from build123d import *

# Parameters (mm, degrees)
F0_W      = 1200
F0_H      = 145
F1_DEPTH  = 22
F0_H_2    = 100
F2_W      = 145
F2_H      = 655
F2_H_2    = 145
F3_DEPTH  = 22
F4_W      = 145
F4_H      = 100
F6_DEPTH  = 78
F4_H_2    = 145
F5_W      = 145
F5_H      = 145
F5_H_2    = 100
F7_W      = 145
F7_H      = 100
F7_W_2    = 1055
F8_DEPTH  = 22
F7_W_3    = 1200
F7_H_2    = 145
F10_SIZE  = 15
F11_W     = 527.5
F11_H     = 145
F12_DEPTH = 211


# Not quite as in the source:
# - a feature names something its author has since deleted; it is built from what else it names


with BuildPart() as f1:
    # F0 (on Top) → F1 (new body)
    with BuildSketch(Plane.XY):
        with Locations((0, 327.5)):
            Rectangle(F0_W, F0_H)
    extrude(amount=-F1_DEPTH)


with BuildPart() as f1b:
    # F0 (on Top) → F1, piece 2 (new body)
    with BuildSketch(Plane.XY):
        with Locations((0, 163.75)):
            Rectangle(F0_W, F0_H_2)
    extrude(amount=-F1_DEPTH)


with BuildPart() as f1c:
    # F0 (on Top) → F1, piece 3 (new body)
    with BuildSketch(Plane.XY):
        Rectangle(F0_W, F0_H)
    extrude(amount=-F1_DEPTH)


with BuildPart() as f1d:
    # F0 (on Top) → F1, piece 4 (new body)
    with BuildSketch(Plane.XY):
        with Locations((0, -163.75)):
            Rectangle(F0_W, F0_H_2)
    extrude(amount=-F1_DEPTH)


with BuildPart() as f1e:
    # F0 (on Top) → F1, piece 5 (new body)
    with BuildSketch(Plane.XY):
        with Locations((0, -327.5)):
            Rectangle(F0_W, F0_H)
    extrude(amount=-F1_DEPTH)


with BuildPart() as f3:
    # F2 (on face) → F3 (new body)
    with BuildSketch(Plane(origin=(0, 0, -22), x_dir=(1, 0, 0), z_dir=(0, 0, -1))):
        with Locations((-527.5, -72.5)):
            Rectangle(F2_W, F2_H)
        with Locations((-527.5, 327.5)):
            Rectangle(F2_W, F2_H_2)
    extrude(amount=F3_DEPTH)


with BuildPart() as f3b:
    # F2 (on face) → F3, piece 2 (new body)
    with BuildSketch(Plane(origin=(0, 0, -22), x_dir=(1, 0, 0), z_dir=(0, 0, -1))):
        with Locations((0, 327.5)):
            Rectangle(F2_W, F2_H_2)
        with Locations((0, -72.5)):
            Rectangle(F2_W, F2_H)
    extrude(amount=F3_DEPTH)


with BuildPart() as f3c:
    # F2 (on face) → F3, piece 3 (new body)
    with BuildSketch(Plane(origin=(0, 0, -22), x_dir=(1, 0, 0), z_dir=(0, 0, -1))):
        with Locations((527.5, 327.5)):
            Rectangle(F2_W, F2_H_2)
        with Locations((527.5, -72.5)):
            Rectangle(F2_W, F2_H)
    extrude(amount=F3_DEPTH)


with BuildPart() as f6:
    # F4 (on face) → F6 (new body)
    with BuildSketch(Plane(origin=(0, 0, -44), x_dir=(1, 0, 0), z_dir=(0, 0, -1))):
        with Locations((-527.5, -350)):
            Rectangle(F4_W, F4_H)
    extrude(amount=F6_DEPTH)


with BuildPart() as f6b:
    # F4 (on face) → F6, piece 2 (new body)
    with BuildSketch(Plane(origin=(0, 0, -44), x_dir=(1, 0, 0), z_dir=(0, 0, -1))):
        with Locations((-527.5, 350)):
            Rectangle(F4_W, F4_H)
    extrude(amount=F6_DEPTH)


with BuildPart() as f6c:
    # F4 (on face) → F6, piece 3 (new body)
    with BuildSketch(Plane(origin=(0, 0, -44), x_dir=(1, 0, 0), z_dir=(0, 0, -1))):
        with Locations((527.5, -350)):
            Rectangle(F4_W, F4_H)
    extrude(amount=F6_DEPTH)


with BuildPart() as f6d:
    # F4 (on face) → F6, piece 4 (new body)
    with BuildSketch(Plane(origin=(0, 0, -44), x_dir=(1, 0, 0), z_dir=(0, 0, -1))):
        with Locations((527.5, 0)):
            Rectangle(F4_W, F4_H_2)
    extrude(amount=F6_DEPTH)


with BuildPart() as f6e:
    # F4 (on face) → F6, piece 5 (new body)
    with BuildSketch(Plane(origin=(0, 0, -44), x_dir=(1, 0, 0), z_dir=(0, 0, -1))):
        with Locations((527.5, 350)):
            Rectangle(F4_W, F4_H)
    extrude(amount=F6_DEPTH)


with BuildPart() as f6f:
    # F4 (on face) → F6, piece 6 (new body)
    with BuildSketch(Plane(origin=(0, 0, -44), x_dir=(1, 0, 0), z_dir=(0, 0, -1))):
        with Locations((-527.5, 0)):
            Rectangle(F4_W, F4_H_2)
    extrude(amount=F6_DEPTH)


with BuildPart() as f6g:
    # F5 (on face) → F6, piece 7 (new body)
    with BuildSketch(Plane(origin=(0, 0, -44), x_dir=(1, 0, 0), z_dir=(0, 0, -1))):
        Rectangle(F5_W, F5_H)
    extrude(amount=F6_DEPTH)


with BuildPart() as f6h:
    # F5 (on face) → F6, piece 8 (new body)
    with BuildSketch(Plane(origin=(0, 0, -44), x_dir=(1, 0, 0), z_dir=(0, 0, -1))):
        with Locations((0, 350)):
            Rectangle(F5_W, F5_H_2)
    extrude(amount=F6_DEPTH)


with BuildPart() as f6i:
    # F5 (on face) → F6, piece 9 (new body)
    with BuildSketch(Plane(origin=(0, 0, -44), x_dir=(1, 0, 0), z_dir=(0, 0, -1))):
        with Locations((0, -350)):
            Rectangle(F5_W, F5_H_2)
    extrude(amount=F6_DEPTH)


with BuildPart() as f8:
    # F7 (on face) → F8 (new body)
    with BuildSketch(Plane(origin=(0, 0, -122), x_dir=(1, 0, 0), z_dir=(0, 0, -1))):
        with Locations((-527.5, -350)):
            Rectangle(F7_W, F7_H)
        with Locations((72.5, -350)):
            Rectangle(F7_W_2, F7_H)
    extrude(amount=F8_DEPTH)


with BuildPart() as f8b:
    # F7 (on face) → F8, piece 2 (new body)
    with BuildSketch(Plane(origin=(0, 0, -122), x_dir=(1, 0, 0), z_dir=(0, 0, -1))):
        Rectangle(F7_W_3, F7_H_2)
    extrude(amount=F8_DEPTH)


with BuildPart() as f8c:
    # F7 (on face) → F8, piece 3 (new body)
    with BuildSketch(Plane(origin=(0, 0, -122), x_dir=(1, 0, 0), z_dir=(0, 0, -1))):
        with Locations((0, 350)):
            Rectangle(F7_W_3, F7_H)
    extrude(amount=F8_DEPTH)


with BuildPart() as f3c_1:
    add(f3c.part)

    # F9: union F3b, F3, F1, F1b, F1e, F1d, F1c, F6, F6b, F6d, F6f, F8b, F8c, F6e, F6c, F8, F6i, F6g, F6h
    add(f3b.part)
    add(f3.part)
    add(f1.part)
    add(f1b.part)
    add(f1e.part)
    add(f1d.part)
    add(f1c.part)
    add(f6.part)
    add(f6b.part)
    add(f6d.part)
    add(f6f.part)
    add(f8b.part)
    add(f8c.part)
    add(f6e.part)
    add(f6c.part)
    add(f8.part)
    add(f6i.part)
    add(f6g.part)
    add(f6h.part)

    # F10
    f10_edges = [f3c_1.edges().sort_by_distance(p)[0] for p in [
        (-600, -400, -72),
        (600, -400, -72),
        (600, 400, -72),
        (-600, 400, -72),
    ]]
    chamfer(f10_edges, length=F10_SIZE)

    # F11 (on face) → F12 (cut)
    with BuildSketch(Plane(origin=(0, 0, -144), x_dir=(1, 0, 0), z_dir=(0, 0, -1))):
        with Locations((336.25, 0)):
            Rectangle(F11_W, F11_H)
        Polygon((672.5, -500), (672.5, 300), (72.5, 300), (72.5, 72.5), (600, 72.5), (600, -72.5), (72.5, -72.5), (72.5, -500), align=None)
    extrude(amount=-F12_DEPTH, mode=Mode.SUBTRACT)


solid = f3c_1.part
Read the model definition and answer for the solid it produces. Units are mm, in the model's axes. A direction names the side the tool comes from. Coordinates: 2 decimals unless noted, no trailing zeros. Loops run counter-clockwise (first coordinate to the right, second up) from the corner with the lowest first, then second, coordinate; pieces in that order, holes last.
Q1. The part is cut by section C-C on y = 320. Write down the section's boundary in (x, z), and give its area (3 significant figures).
Q2. The mould has two halves that part along Z. Classify faces 1 (the face through (-8, -400, -71)), 2 (the face through (261, -351, -122)), 3 (the face through (-8, -343, 0)), 4 (the face through (261, -349, -22)): +Z half, -Z half, draft (parallel to the pull), parting line (faces both ways), or undercut.
Q3. The part is cut by section B-B on z = -94. Give the number of separate pieces and of enclosed holes in the cut face, and give its area (3 significant figures).
Q4. The part is cut by section A-A on x = 434. Write down the section's boundary in (y, z), and give its area (3 significant figures).
Q5. Consider probe 1 along Y at (x, z) = (-118, -136); probe 2 along Y at (x, z) = (-445, -16); probe 3 along X at (y, z) = (-360, -38.5). Determine where each line is inside the solid, lowest interval first.
Q6. Which of the six approach directions +Z, -Z, +X, -X, +Y, -Y give full straight-line access (tool end or side, diameter ignored) to faces 5 (the face through (-1, -93, -22)), 6 (the face through (-266, 1, -22)), 7 (the face through (142, -300, -137))?
Q7. This flat-tipped pin is pushed along its axis until it touches: pin 1 Ø12.5 at (x, y) = (34, -237.5) entering from +Z. Where does it stop, or does it pass through?
Results below:
1. outline: (-600, -144) - (72.5, -144) - (72.5, 0) - (-600, 0) - close; hole (-455, -122) - (-72.5, -122) - (-72.5, -22) - (-455, -22) - close
1. area: 58,600 mm2
2. face 1: draft
2. face 2: undercut
2. face 3: +Z half
2. face 4: undercut
3. separate pieces: 7
3. enclosed holes: 0
3. area: 114,000 mm2
4. outline: (-400, -144) - (-300, -144) - (-300, -122) - (-400, -122) - close; (-400, -22) - (-300, -22) - (-300, 0) - (-400, 0) - close
4. area: 4,400 mm2
5. probe 1: y = -400 to -300, -72.5 to 72.5, 300 to 400
5. probe 2: y = -400 to -255, -213.75 to -113.75, -72.5 to 72.5, 113.75 to 213.75, 255 to 400
5. probe 3: x = -600 to -455, -72.5 to 72.5, 455 to 600
6. face 5: +Z, +X, -X
6. face 6: +Y, -Y
6. face 7: -Z, +X
7. pin 1: stops at z = -22
